from build123d import *

# Parameters (mm, degrees)
ESQUISSE1_W        = 18
ESQUISSE1_H        = 8
BOSS_EXTRU_1_DEPTH = 5
ESQUISSE2_W        = 6.4
ESQUISSE2_H        = 2
BOSS_EXTRU_2_DEPTH = 5


with BuildPart() as part:
    # Esquisse1 → Boss.-Extru.1 (new body)
    with BuildSketch(Plane(origin=(0, 0, 0), x_dir=(1, 0, 0), z_dir=(0, 1, 0))):
        Rectangle(ESQUISSE1_W, ESQUISSE1_H)
    extrude(amount=BOSS_EXTRU_1_DEPTH)

    # Esquisse2 → Boss.-Extru.2 (add)
    with BuildSketch(Plane.XY.offset(4)):
        with Locations((0, 1)):
            Rectangle(ESQUISSE2_W, ESQUISSE2_H)
    extrude(amount=BOSS_EXTRU_2_DEPTH)


solid = part.part
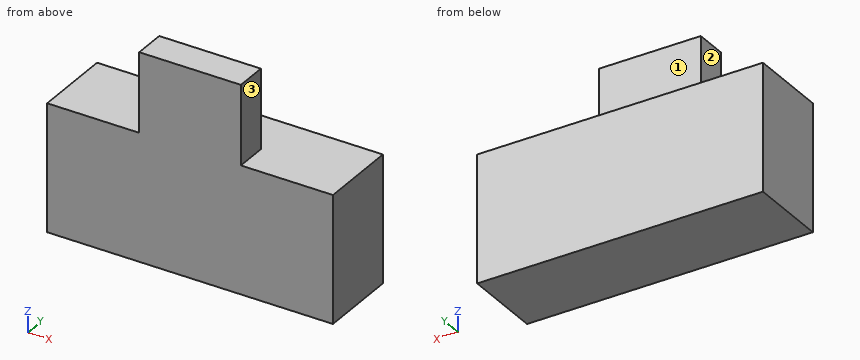
For this review, take the finished solid that the model builds, in its own axes (mm). Face numbers are marked on the shaded views. A direction names the side the tool comes from. Round coordinates to 2 decimals unless told otherwise and drop trailing zeros. Order: outer loops, then holes, each group sorted by start corner. A loop starts at its lowest first (then second) coordinate and runs counter-clockwise, first axis right, second up. Notation, with made-up numbers: (0.5, 63) -> (54.5, 63) arc R4 ccw to (54.5, 68) -> close; hole circle Ø3 at (60.5, -30.75). An arc over 180 degrees is marked (long way). Put each result on its own line as item: value.
Q1. Add section A-A on y = 1.25. Write out the cut boundary in (x, z).
Check result:
outline: (-9, -4) -> (9, -4) -> (9, 4) -> (3.2, 4) -> (3.2, 9) -> (-3.2, 9) -> (-3.2, 4) -> (-9, 4) -> close
Q2. Machinability: for the marked faces 1, 2 and 3, which of the approach directions +Z, -Z, +X, -X, +Y, -Y give a long, thin tool a straight path to every point of the face, cutting with its end or side? Answer none if there is none.
Check result:
face 1: +Z, +X, -X, +Y
face 2: +Z, -X, +Y, -Y
face 3: +Z, +X, +Y, -Y
Q3. Add section D-D on x = 4. Write out the cut boundary in (y, z), plus the area to 3 significant figures.
Check result:
outline: (0, -4) -> (5, -4) -> (5, 4) -> (0, 4) -> close
area: 40.0 mm2
Q4. For probe 1 along X at (y, z) = (0.7, 4.75); probe 2 along Y at (x, z) = (-0.75, 6.5); probe 3 along Z at (x, y) = (-5.5, 3.25), list the stretches that pass through material, from the lowest coordinate up. Write a range as [from, to].
Check result:
probe 1: [-3.2, 3.2]
probe 2: [0, 2]
probe 3: [-4, 4]
Q5. Add section C-C on z = 6.75. Write out the cut boundary in (x, y), plus the area to 3 significant figures.
Check result:
outline: (-3.2, 0) -> (3.2, 0) -> (3.2, 2) -> (-3.2, 2) -> close
area: 12.8 mm2
Q6. Add section B-B on x = -2. Write out the cut boundary in (y, z).
Check result:
outline: (0, -4) -> (5, -4) -> (5, 4) -> (2, 4) -> (2, 9) -> (0, 9) -> close
Q7. Insertion check: pin 1 Ø2 at (y, z) = (0.5, 7) entering from -X; pin 2 Ø1 at (y, z) = (0.5, 5.5) entering from +X. Each pin has a flat end and moves straight along its axis. Give the tip position at first contact, or say it passes through.
Check result:
pin 1: x = -3.2
pin 2: x = 3.2
